The figure shows three views and two pictorial views of one solid part (mm, origin at its lowest corner). Answer the questions. Coordinates: 2 decimals unless noted, no trailing zeros. Write each loop counter-clockwise with the first axis right and the second up, starting at its lowest first coordinate (ties: lowest second). Pieces come first, ordered by that corner, then holes. Notation, with made-up numbers: M 68.25,48 L 84.25,48 A18 ccw 84.25,62 Z; hole C -16,-20 d8. An arc over 180 degrees is marked long. Use a Markdown table: item, result. Add a question column.
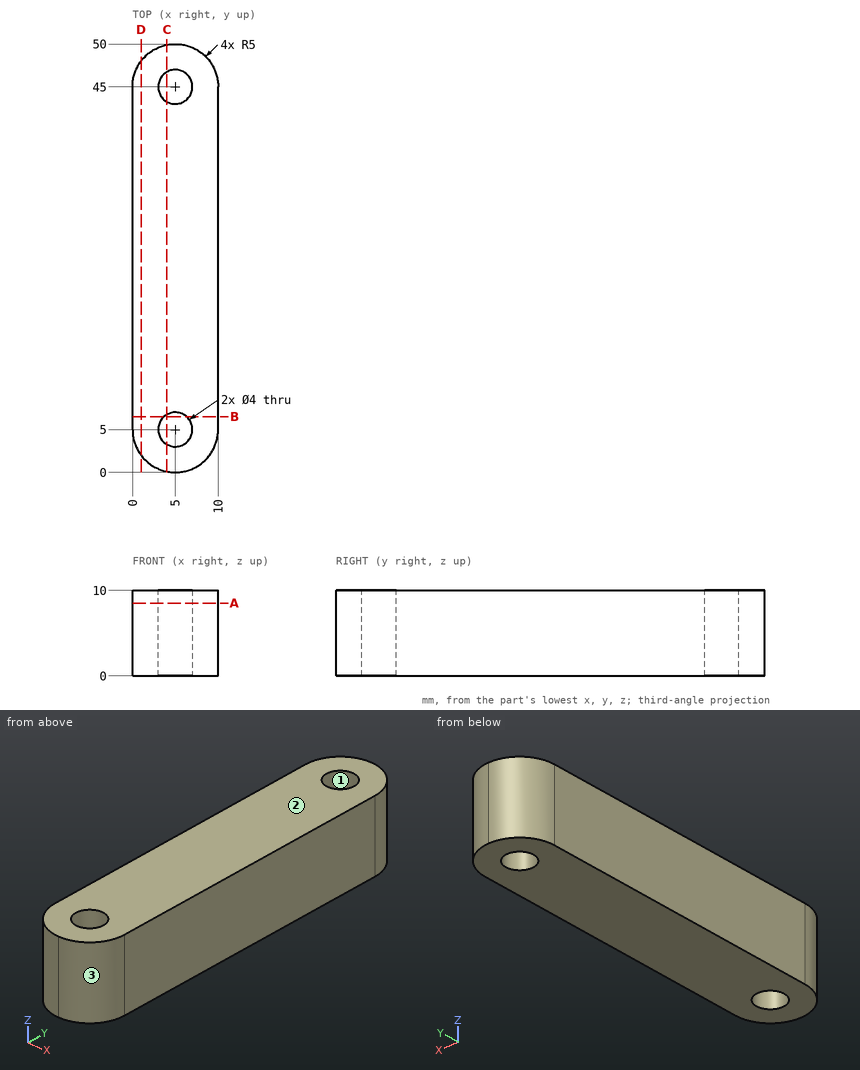
Item 1: Determine the mould class of the marked faces 1, 2 and 3 for opening direction Y: pulls with the +Y half, pulls with the -Y half, needs draft (parallel to the pull), parting line crosses it, or undercut.
Item 2: Consider probe 1 along Y at (x, z) = (5, 3); probe 2 along Y at (x, z) = (3.5, 6.5); probe 3 along Y at (x, z) = (9, 4.25). Determine where each line is inside the solid, lowest interval first.
Item 3: Find section C-C on x = 4. Give the vertices of the cut face in (y, z).
Item 4: Find section B-B on y = 6.5. Give the vertices of the cut face in (x, z).
Item 5: Find section A-A on z = 8.5. Count the separate pieces of the cut face and the enclosed holes in it, then the cut area to 3 significant figures.
Item 6: Each of these flat-tipped pins is pushed along its axis until it touches: pin 1 (2.5 mm diameter, centred on x = 5, y = 45, fed in from +Z); pin 2 (3 mm diameter, centred on y = 27, z = 3.5, fed in from -X). Where does it stop, or does it pass through?
Item 7: Find section D-D on x = 1. Give the vertices of the cut face in (y, z), then the cut area to 3 significant figures.
Geometry says:
| question | item | result |
|---|---|---|
| 1 | face 1 | undercut |
| 1 | face 2 | needs draft |
| 1 | face 3 | pulls with the -Y half |
| 2 | probe 1 | y = 0 to 3, 7 to 43, 47 to 50 |
| 2 | probe 2 | y = 0.23 to 3.68, 6.32 to 43.68, 46.32 to 49.77 |
| 2 | probe 3 | y = 2 to 48 |
| 3 | outline | M 0.1,0 L 3.27,0 L 3.27,10 L 0.1,10 Z; M 6.73,0 L 43.27,0 L 43.27,10 L 6.73,10 Z; M 46.73,0 L 49.9,0 L 49.9,10 L 46.73,10 Z |
| 4 | outline | M 0,0 L 3.68,0 L 3.68,10 L 0,10 Z; M 6.32,0 L 10,0 L 10,10 L 6.32,10 Z |
| 5 | separate pieces | 1 |
| 5 | enclosed holes | 2 |
| 5 | area | 453 mm2 |
| 6 | pin 1 | passes through |
| 6 | pin 2 | stops at x = 0 |
| 7 | outline | M 2,0 L 48,0 L 48,10 L 2,10 Z |
| 7 | area | 460 mm2 |
